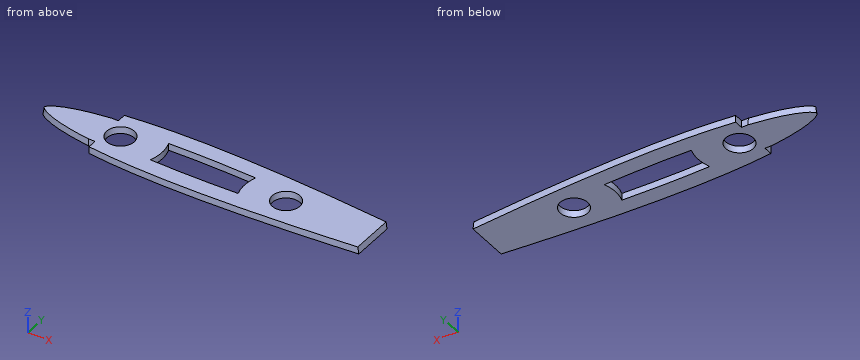
```python
from build123d import *

# Parameters (mm, degrees)
BOSS_EXTRUDE1_DEPTH     = 3.175
SKETCH2_R               = 6.35
CUT_EXTRUDE1_DEPTH      = 3.175
CUT_EXTRUDE2_DEPTH      = 15.229125104
CUT_EXTRUDE2_DEPTH_BACK = 15.229125104
CUT_EXTRUDE3_DEPTH      = 7.62


with BuildPart() as part:
    # Sketch1 → Boss-Extrude1 (new body)
    with BuildSketch(Plane.XY):
        with BuildLine():
            add(Edge.make_bspline(
                [(237.0836, 0.298725336), (236.995594177, 0.372475408), (236.426976915, 0.302841036), (235.414414738, 0.587878253), (233.557510406, 0.764057302), (231.055978259, 1.142159154), (227.833630131, 1.564095564), (223.947681725, 2.084112793), (219.408243114, 2.671942868), (214.248186401, 3.326415443), (208.497669056, 4.03606524), (202.192664292, 4.791288168), (195.371926847, 5.582717259), (188.077459081, 6.399577403), (180.354259346, 7.2318954), (172.249998357, 8.069333754), (163.814621862, 8.901083193), (155.10015976, 9.715468455), (146.160279484, 10.50179834), (137.050196099, 11.246926821), (127.825887085, 11.938704549), (118.544307176, 12.564288117), (109.262643889, 13.110597113), (100.038037253, 13.563829729), (90.927458146, 13.911900095), (81.986813488, 14.143452851), (73.27135464, 14.247178081), (64.83463449, 14.214844108), (56.728667619, 14.040205364), (49.003349951, 13.718834947), (41.706232299, 13.249892202), (34.882163012, 12.634788148), (28.572900537, 11.878326773), (22.816901851, 10.986944444), (17.649046914, 9.969950888), (13.099625234, 8.838845522), (9.194488598, 7.604658034), (5.953477664, 6.278883166), (3.386928106, 4.870490409), (1.49878923, 3.376700029), (0.289451642, 1.761373844), (-0.134894757, 0), (0.289451642, -1.761373844), (1.49878923, -3.376700029), (3.386928106, -4.870490409), (5.953477664, -6.278883166), (9.194488598, -7.604658034), (13.099625234, -8.838845522), (17.649046914, -9.969950888), (22.816901851, -10.986944444), (28.572900537, -11.878326773), (34.882163012, -12.634788148), (41.706232299, -13.249892202), (49.003349951, -13.718834947), (56.728667619, -14.040205364), (64.83463449, -14.214844108), (73.27135464, -14.247178081), (81.986813488, -14.143452851), (90.927458146, -13.911900095), (100.038037253, -13.563829729), (109.262643889, -13.110597113), (118.544307176, -12.564288117), (127.825887085, -11.938704549), (137.050196099, -11.246926821), (146.160279484, -10.50179834), (155.10015976, -9.715468455), (163.814621862, -8.901083193), (172.249998357, -8.069333754), (180.354259346, -7.2318954), (188.077459081, -6.399577403), (195.371926847, -5.582717259), (202.192664292, -4.791288168), (208.497669056, -4.03606524), (214.248186401, -3.326415443), (219.408243114, -2.671942868), (223.947681725, -2.084112793), (227.833630131, -1.564095564), (231.055978259, -1.142159154), (233.557510406, -0.764057302), (235.414414738, -0.587878253), (236.426976915, -0.302841036), (237.226122795, -0.400706552), (237.226122795, 0.179289302), (237.0836, 0.298725336)],
                knots=[0, 0, 0, 0, 0.000762215, 0.003044706, 0.006832246, 0.012101176, 0.018817536, 0.026939455, 0.036414848, 0.047184629, 0.059180413, 0.072327874, 0.086544061, 0.10174058, 0.117823336, 0.134691452, 0.152240154, 0.17036129, 0.188941008, 0.207865435, 0.227016078, 0.246275696, 0.265524943, 0.284644966, 0.303520118, 0.322034575, 0.340078353, 0.357542593, 0.374325482, 0.390329891, 0.40546389, 0.419643801, 0.432793371, 0.444843817, 0.455737921, 0.465428653, 0.47388632, 0.481101634, 0.487101684, 0.491975368, 0.495930678, 0.499382808, 0.502834938, 0.506790248, 0.511663932, 0.517663982, 0.524879296, 0.533336963, 0.543027695, 0.553921799, 0.565972245, 0.579121815, 0.593301726, 0.608435725, 0.624440134, 0.641223023, 0.658687263, 0.676731041, 0.695245498, 0.71412065, 0.733240673, 0.75248992, 0.771749538, 0.790900181, 0.809824608, 0.828404326, 0.846525462, 0.864074164, 0.88094228, 0.897025036, 0.912221555, 0.926437743, 0.939585203, 0.951580988, 0.962350768, 0.971826161, 0.979948081, 0.98666444, 0.991933371, 0.99572091, 0.998003402, 0.998765616, 1, 1, 1, 1], degree=3))
        make_face()
    extrude(amount=BOSS_EXTRUDE1_DEPTH)

    # Sketch2 → Cut-Extrude1 (cut)
    with BuildSketch(Plane.XY.offset(3.175)):
        with Locations((38.1, 0)):
            Circle(SKETCH2_R)
        with Locations((114.3, 0)):
            Circle(SKETCH2_R)
    extrude(amount=-CUT_EXTRUDE1_DEPTH, mode=Mode.SUBTRACT)

    # Sketch3 → Cut-Extrude2 (cut, two sides)
    with BuildSketch(Plane(origin=(0, 0, 0), x_dir=(1, 0, 0), z_dir=(0, 1, 0))) as cut_extrude2_sk:
        Polygon((154.274292451, 0), (153.827643764, -3.175), (237.190492096, -3.175), (237.190492096, 0), align=None)
    extrude(amount=CUT_EXTRUDE2_DEPTH, mode=Mode.SUBTRACT)
    extrude(cut_extrude2_sk.sketch, amount=-CUT_EXTRUDE2_DEPTH_BACK, mode=Mode.SUBTRACT)

    # Sketch6 → Cut-Loft1 section 0
    with BuildSketch(Plane.XY.offset(3.175)):
        with BuildLine():
            Line((31.75, 8.076408981), (31.75, 11.683250037))
            Line((31.75, 11.683250037), (31.75, 18.395885889))
            Line((31.75, 18.395885889), (-8.998418256, 14.186873402))
            Line((-8.998418256, 14.186873402), (-8.032236021, -19.061162304))
            Line((-8.032236021, -19.061162304), (31.75, -17.664488176))
            Line((31.75, -17.664488176), (31.75, -11.683250037))
            Line((31.75, -11.683250037), (31.75, -8.076408982))
            Line((31.75, -8.076408982), (28.702, -8.076408982))
            add(Edge.make_bspline(
                [(28.702, 8.076408981), (28.062019842, 7.997428017), (26.781360323, 7.83190678), (24.863238423, 7.559576486), (22.952864289, 7.261817641), (21.053229662, 6.936585888), (19.16878625, 6.582266966), (17.301352642, 6.194891801), (15.452394184, 5.770523851), (13.933846318, 5.382610192), (12.734807014, 5.049324169), (11.845778194, 4.787008043), (10.968295358, 4.511299981), (10.104114856, 4.221132537), (9.254625692, 3.915388001), (8.425053114, 3.594578064), (7.620756036, 3.259288164), (6.846465326, 2.908873288), (6.109521351, 2.54404498), (5.415085904, 2.161886878), (4.771732283, 1.761162286), (4.200618093, 1.360175223), (3.806381168, 1.039757171), (3.546177048, 0.785599694), (3.383920596, 0.598121849), (3.254767765, 0.412598836), (3.174243399, 0.254294099), (3.130379566, 0.1138318), (3.117983008, 3.16e-07), (3.130380113, -0.113832551), (3.174242347, -0.254293127), (3.254769825, -0.41260053), (3.383916396, -0.598118576), (3.546175023, -0.785598191), (3.806491944, -1.039841143), (4.20055318, -1.360126113), (4.77176705, -1.761188423), (5.41506381, -2.161870561), (6.109540545, -2.544058683), (6.846443726, -2.908858743), (7.620785984, -3.259307593), (8.424980153, -3.594531648), (9.25458748, -3.915363972), (10.104136109, -4.221145998), (10.968310445, -4.511309444), (11.845765894, -4.787000103), (12.734797781, -5.049319704), (13.933888924, -5.382621972), (15.4523656, -5.770516248), (17.301363518, -6.194894525), (19.168788744, -6.582267832), (21.053210036, -6.936580559), (22.952903047, -7.261827785), (24.863140664, -7.559551063), (26.781311277, -7.831894211), (28.062019842, -7.997428017), (28.702, -8.076408982)],
                knots=[0, 0, 0, 0, 0.03125, 0.0625, 0.09375, 0.125, 0.15625, 0.1875, 0.21875, 0.25, 0.265625, 0.28125, 0.296875, 0.3125, 0.328125, 0.34375, 0.359375, 0.375, 0.390625, 0.40625, 0.421875, 0.4375, 0.453125, 0.4609375, 0.46875, 0.4765625, 0.484375, 0.4921875, 0.5, 0.5078125, 0.515625, 0.5234375, 0.53125, 0.5390625, 0.546875, 0.5625, 0.578125, 0.59375, 0.609375, 0.625, 0.640625, 0.65625, 0.671875, 0.6875, 0.703125, 0.71875, 0.734375, 0.75, 0.78125, 0.8125, 0.84375, 0.875, 0.90625, 0.9375, 0.96875, 1, 1, 1, 1], degree=3))
            Line((28.702, 8.076408981), (31.75, 8.076408981))
        make_face()
    # Sketch5 → Cut-Loft1 section 1
    with BuildSketch(Plane(origin=(0, 0, 0), x_dir=(-1, 0, 0), z_dir=(0, 0, -1))):
        with BuildLine():
            Line((-31.75, -11.773629767), (-31.75, -8.172962021))
            Line((-31.75, -8.172962021), (-28.702, -8.172962021))
            add(Edge.make_bspline(
                [(-28.702, 8.17296202), (-28.04991232, 8.094156153), (-26.745045473, 7.928885379), (-24.790625464, 7.656596528), (-22.843952156, 7.358509388), (-20.907993005, 7.032534185), (-18.987137813, 6.677003012), (-17.083250909, 6.287895965), (-15.197789513, 5.861217163), (-13.648800631, 5.470809812), (-12.425346674, 5.135128731), (-11.518003122, 4.870795331), (-10.622183079, 4.592820857), (-9.739660488, 4.300116815), (-8.871825969, 3.991542258), (-8.023884998, 3.667528855), (-7.201182529, 3.328585226), (-6.408478992, 2.973975846), (-5.653156453, 2.604323149), (-4.940474095, 2.216549268), (-4.279203879, 1.809302193), (-3.690786556, 1.400484278), (-3.283034517, 1.072052932), (-3.013354261, 0.810752852), (-2.845020129, 0.61774711), (-2.710958875, 0.426579544), (-2.627372313, 0.263337315), (-2.58177414, 0.117962243), (-2.568858472, 3.28e-07), (-2.581774708, -0.117963026), (-2.627371214, -0.263336298), (-2.710961028, -0.426581314), (-2.845015751, -0.617743699), (-3.01335214, -0.810751279), (-3.283150094, -1.072140545), (-3.690718878, -1.400433069), (-4.27924005, -1.809329397), (-4.940451244, -2.216532371), (-5.653176086, -2.604337198), (-6.408457303, -2.973961207), (-7.201212263, -3.32860454), (-8.023812968, -3.667483017), (-8.871788374, -3.991518624), (-9.739681391, -4.300130053), (-10.622197985, -4.592830206), (-11.517990976, -4.870787488), (-12.425337452, -5.135124325), (-13.648844495, -5.470821714), (-15.197759965, -5.861209465), (-17.083262354, -6.287898751), (-18.987139884, -6.677003815), (-20.907973868, -7.032528958), (-22.843990245, -7.358519372), (-24.790529171, -7.656571477), (-26.744997097, -7.928872987), (-28.04991232, -8.094156153), (-28.702, -8.172962021)],
                knots=[0, 0, 0, 0, 0.03125, 0.0625, 0.09375, 0.125, 0.15625, 0.1875, 0.21875, 0.25, 0.265625, 0.28125, 0.296875, 0.3125, 0.328125, 0.34375, 0.359375, 0.375, 0.390625, 0.40625, 0.421875, 0.4375, 0.453125, 0.4609375, 0.46875, 0.4765625, 0.484375, 0.4921875, 0.5, 0.5078125, 0.515625, 0.5234375, 0.53125, 0.5390625, 0.546875, 0.5625, 0.578125, 0.59375, 0.609375, 0.625, 0.640625, 0.65625, 0.671875, 0.6875, 0.703125, 0.71875, 0.734375, 0.75, 0.78125, 0.8125, 0.84375, 0.875, 0.90625, 0.9375, 0.96875, 1, 1, 1, 1], degree=3))
            Line((-28.702, 8.17296202), (-31.75, 8.17296202))
            Line((-31.75, 8.17296202), (-31.75, 11.773629767))
            Line((-31.75, 11.773629767), (-31.75, 14.858712547))
            Line((-31.75, 14.858712547), (1.815959964, 11.773629767))
            Line((1.815959964, 11.773629767), (0.454850161, -12.744594259))
            Line((0.454850161, -12.744594259), (-31.75, -15.902369002))
            Line((-31.75, -15.902369002), (-31.75, -11.773629767))
        make_face()
    loft(mode=Mode.SUBTRACT)

    # Sketch7 → Cut-Extrude3 (cut)
    with BuildSketch(Plane.XY.offset(3.175)):
        with BuildLine():
            ThreePointArc((56.054224621, -6.367756139), (57.15, 0), (56.054224621, 6.367756139))
            add(Edge.make_bspline(
                [(96.245779506, 6.07845559), (93.861405197, 6.172308422), (91.477846396, 6.255305153), (84.344598798, 6.468290826), (79.598726683, 6.562324228), (70.121487659, 6.629056545), (65.389943722, 6.602176751), (59.131701158, 6.462519155), (57.592019112, 6.419793098), (56.054224621, 6.367756139)],
                knots=[0.437309704, 0.437309704, 0.437309704, 0.437309704, 0.5, 0.5, 0.625, 0.625, 0.75, 0.75, 0.790835922, 0.790835922, 0.790835922, 0.790835922], degree=3))
            ThreePointArc((96.245779506, 6.07845559), (95.25, 0), (96.245779506, -6.07845559))
            add(Edge.make_bspline(
                [(56.054224621, -6.367756139), (57.592019112, -6.419793098), (59.131701158, -6.462519155), (65.389943722, -6.602176751), (70.121487659, -6.629056545), (79.598726683, -6.562324228), (84.344598798, -6.468290826), (91.477846396, -6.255305153), (93.861405197, -6.172308422), (96.245779506, -6.07845559)],
                knots=[0.209164078, 0.209164078, 0.209164078, 0.209164078, 0.25, 0.25, 0.375, 0.375, 0.5, 0.5, 0.562690296, 0.562690296, 0.562690296, 0.562690296], degree=3))
        make_face()
    extrude(amount=-CUT_EXTRUDE3_DEPTH, mode=Mode.SUBTRACT)


solid = part.part
```
Model file for the job. Use its own axes, mm. Coordinates: 2 decimals unless noted, no trailing zeros. Write item = value, one per line. Start each with the question number.
Item 1: Drop a flat-ended pin along its axis: pin 1 Ø1.5 at (x, y) = (102.5, -10) entering from -Z. Give the stop position or say it passes through.
Item 2: Wall check: probe 1 along X at (y, z) = (-1.75, 2.3); probe 2 along X at (y, z) = (-8.5, 0.2); probe 3 along Y at (x, z) = (82, 1.6). Give the ranges that are in metal, low to high. Write a range as [from, to].
Item 3: Saw through at A-A, the plane y = 0. State how many separate pieces and enclosed holes the cut face has, then the cut area to 3 significant figures.
Answers:
q1.pin_1 = 0
q2.probe_1 = [4.61, 32], [44.2, 57.07], [95.33, 108.2], [120.4, 153.95]
q2.probe_2 = [31.75, 154.25]
q2.probe_3 = [-14.12, -6.5], [6.5, 14.12]
q3.separate_pieces = 4
q3.enclosed_holes = 0
q3.area = 278 mm2
